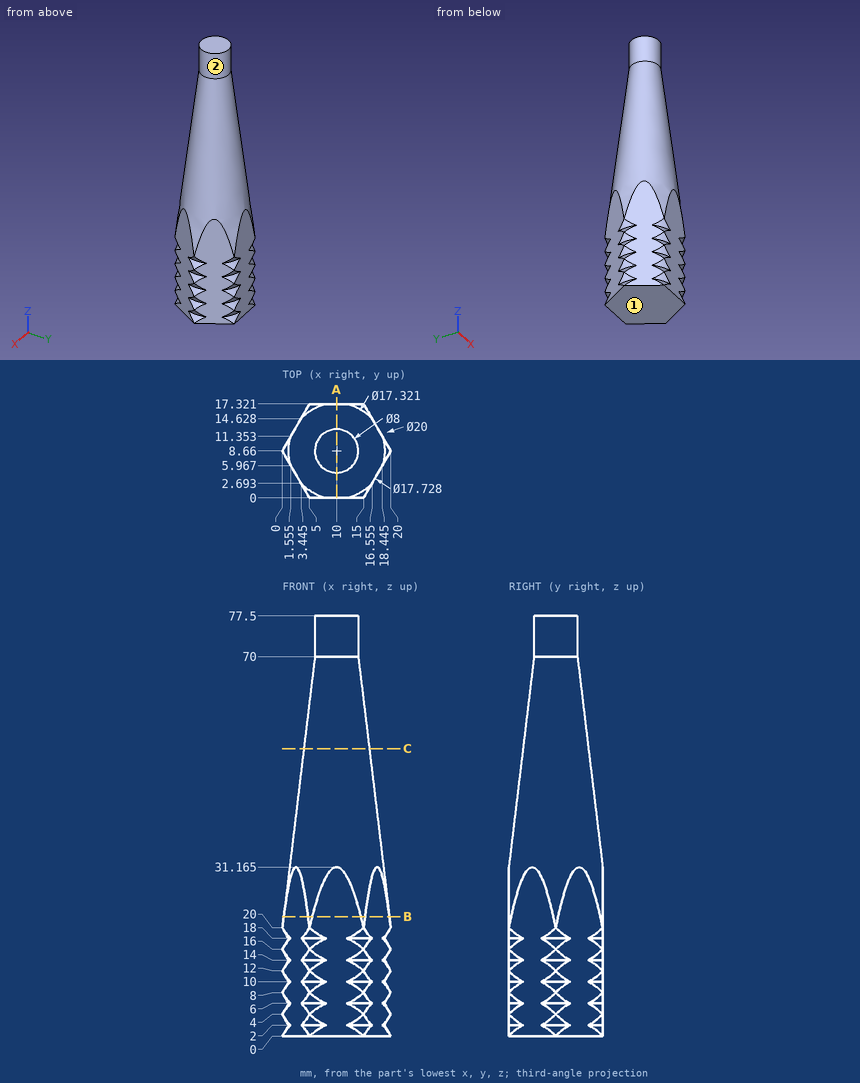
Geometry check sheet. Reference: drawing and pictorial views, mm from the part's lowest x, y, z. A direction names the side the tool comes from. Coordinates: 2 decimals unless noted, no trailing zeros. Write each loop counter-clockwise with the first axis right and the second up, starting at its lowest first coordinate (ties: lowest second). Pieces come first, ordered by that corner, then holes. Notation, with made-up numbers: (-14.75, 21) -> (32.25, 21) arc R13 cw to (32.25, 45) -> close; hole circle Ø9 at (-8.75, 89). An arc over 180 degrees is marked (long way). One line per question, with ' | ' between items.
1. Cross-section at C-C on z = 53. Record the cut outline in (x, y).
Answers:
outline: circle Ø12.08 at (10, 8.66)
2. Cross-section at B-B on z = 22. Record the cut outline in (x, y), and give its area (3 significant figures).
Answers:
outline: (0.25, 8.23) -> (4.75, 0.43) arc R9.76 ccw to (5.5, 0) -> (14.5, 0) arc R9.76 ccw to (15.25, 0.43) -> (19.75, 8.23) arc R9.76 ccw to (19.75, 9.09) -> (15.25, 16.89) arc R9.76 ccw to (14.5, 17.32) -> (5.5, 17.32) arc R9.76 ccw to (4.75, 16.89) -> (0.25, 9.09) arc R9.76 ccw to start | area: 259 mm²
3. Cross-section at A-A on x = 10. Record the cut outline in (y, z) (1 decimal).
Answers:
outline: (0, 0) -> (17.3, 0) -> (17.3, 31.2) -> (12.7, 70) -> (12.7, 77.5) -> (4.7, 77.5) -> (4.7, 70) -> (0, 31.2) -> close
4. Set-up check for the marked faces 1 and 2: record each of +Z, -Z, +X, -X, +Y, -Y from which the full face is reachable in a straight line by a thin tool's end or side.
Answers:
face 1: -Z, +X, -X, +Y, -Y | face 2: +Z
5. Depth check by flat-ended pin: pin 1 Ø10 at (y, z) = (2, 59) entering from +X (1 decimal); pin 2 Ø4 at (y, z) = (10.5, 23) entering from +X (1 decimal); pin 3 Ø2 at (y, z) = (9.5, 59) entering from -X; pin 4 Ø12 at (x, z) = (6.5, 10) entering from -Y. Enter the tip coordinate at first touch or a pass-through.
Answers:
pin 1: stops at x = 15.2 | pin 2: stops at x = 19.8 | pin 3: stops at x = 4.59 | pin 4: stops at y = 0
6. Thickness scan on probe 1 along X at (y, z) = (8.75, 74); probe 2 along Y at (x, z) = (11, 59) (1 decimal); probe 3 along X at (y, z) = (10.75, 13.5) (1 decimal). Record the ranges inside material, lowest first. Write a range as from..to.
Answers:
probe 1: x = 6..14 | probe 2: y = 3.4..13.9 | probe 3: x = 1.2..18.8
